The model under review builds one solid part; all positions refer to its coordinate system, in mm. A direction names the side the tool comes from. Coordinates: 2 decimals unless noted, no trailing zeros. Loops run counter-clockwise (first coordinate to the right, second up) from the corner with the lowest first, then second, coordinate; pieces in that order, holes last. Notation, with made-up numbers: M 73.25,48.5 L 118.25,48.5 A7 ccw 118.25,60.5 Z; hole C 17,83.5 d4. An arc over 180 degrees is marked long. Return JSON: item names as keys, results as strings.
Autodesk Inventor part; units mm, degrees
ref_plane "YZ Plane" through (0, 0, 0) normal (1, 0, 0) x (0, 1, 0)
ref_plane "XZ Plane" through (0, 0, 0) normal (0, 1, 0) x (-1, 0, 0)
ref_plane "XY Plane" through (0, 0, 0) normal (0, 0, 1) x (1, 0, 0)
sketch "Boceto1" plane through (0, 0, 0) normal (0, 0, 1) x (1, 0, 0)
  line L0 (-37.5, 37.5) -> (37.5, 37.5)
  line L1 (37.5, 37.5) -> (37.5, -37.5)
  line L2 (37.5, -37.5) -> (-37.5, -37.5)
  line L3 (-37.5, -37.5) -> (-37.5, 37.5)
  line L4 (34.5, 34.5) -> (-34.5, 34.5)
  line L5 (-34.5, 34.5) -> (-34.5, -34.5)
  line L6 (-34.5, -34.5) -> (34.5, -34.5)
  line L7 (34.5, -34.5) -> (34.5, 34.5)
  point P0 (0, 0)
  dimension "d0" = 75
  dimension "d1" = 75
  dimension "d2" = 3
  dimension "d3" = 37.5
  dimension "d4" = 37.5
extrude "Extrusión1" add sketch "Boceto1" along normal mid plane 2100
equation "\"d0\" = width"
equation "\"d1\" = height"
equation "\"d2\" = t"
equation "\"d5\" = length"
equation "\"width\" = 75"
equation "\"height\" = 75"
equation "\"t\" = 3"
equation "\"length\" = 2100"
properties part number "210 STEEL PROFILE" material "Acero"
1. The part is to be moulded in two halves that separate along X. For faces 3 (the face through (0, -34.5, -15)), 4 (the face through (37.5, 1, -15)), 5 (the face through (-3, -36, 1050)), 6 (the face through (-37.5, -1, -15)), say which applies: released by +X, released by -X, zero draft, split by the parting line, or undercut.
Check values:
{"face 3": "undercut", "face 4": "released by +X", "face 5": "zero draft", "face 6": "released by -X"}
2. To check wall thickness, follow line 1 (Y direction, x = 3, z = 92). State the ranges of the line that lie inside material, in increasing order.
Check values:
{"line 1": "-37.5 to -34.5, 34.5 to 37.5"}
3. Add section C-C on z = 791. Give the boundary of the cut face in (x, y).
Check values:
{"outline": "M -37.5,-37.5 L 37.5,-37.5 L 37.5,37.5 L -37.5,37.5 Z; hole M -34.5,-34.5 L 34.5,-34.5 L 34.5,34.5 L -34.5,34.5 Z"}
4. Add section A-A on y = 16.5. Give the boundary of the cut face in (x, z).
Check values:
{"outline": "M -37.5,-1050 L -34.5,-1050 L -34.5,1050 L -37.5,1050 Z; M 34.5,-1050 L 37.5,-1050 L 37.5,1050 L 34.5,1050 Z"}
5. Machinability: for faces 1 (the face through (-1, 37.5, -15)), 2 (the face through (0, 34.5, -15)), which of the approach directions +Z, -Z, +X, -X, +Y, -Y give a long, thin tool a straight path to every point of the face, cutting with its end or side? Answer none if there is none.
Check values:
{"face 1": "+Z, -Z, +X, -X, +Y", "face 2": "+Z, -Z"}
